Print and shaded views of the part. All mm, measured from the part's lowest x, y and z. A direction names the side the tool comes from. Round coordinates to 2 decimals unless told otherwise and drop trailing zeros. Loops run counter-clockwise (first coordinate to the right, second up) from the corner with the lowest first, then second, coordinate; pieces in that order, holes last. Notation, with made-up numbers: (11, -22) - (31, -22) arc R18 ccw to (31, -9) - close; hole circle Ø2 at (8, 1.5). An arc over 180 degrees is marked (long way). Answer as a JSON object with one key per item and string values.
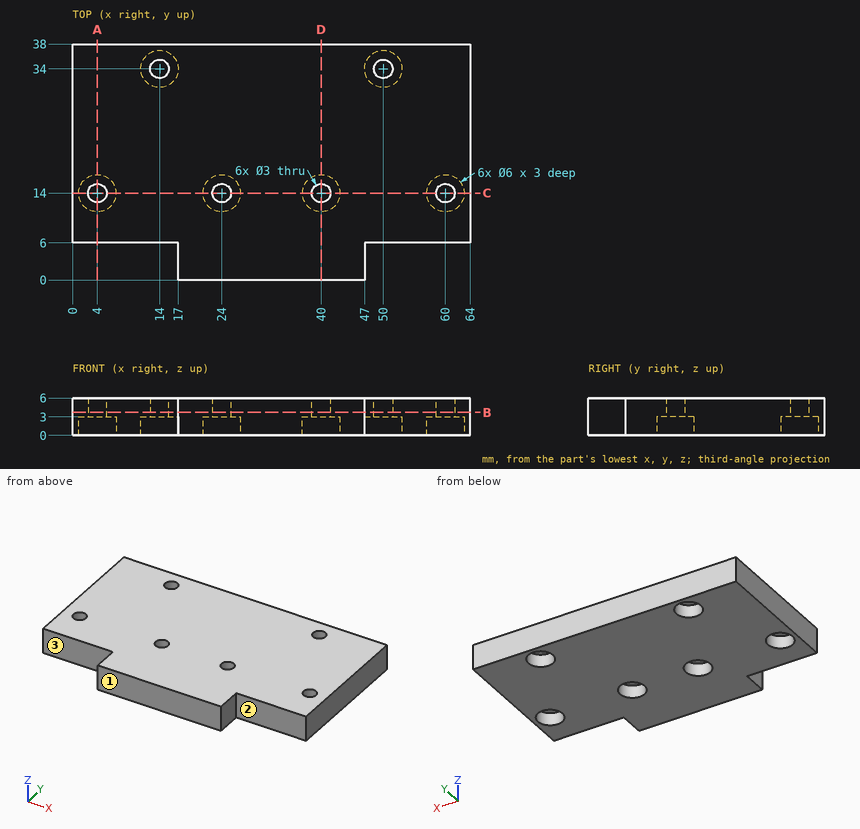
1) Tool access for the marked faces 1, 2 and 3: list every direction of +Z, -Z, +X, -X, +Y, -Y with a clear straight run to the whole face (end or side of a thin tool).
Values follow:
{"face 1": "+Z, -Z, +X, -X, -Y", "face 2": "+Z, -Z, +X, -Y", "face 3": "+Z, -Z, -X, -Y"}
2) Slice it at C-C on y = 14. Count the separate pieces of the cut face and the enclosed holes in it, then the cut area to 3 significant figures.
Values follow:
{"separate pieces": "5", "enclosed holes": "0", "area": "276 mm²"}
3) Drop flat-ended pins along their axis: P1, Ø3, axis at x = 10, z = 3, coming from the -Y side; P2, Ø3.5, axis at x = 50, y = 34, coming from the -Z side. Give the stop position or say it passes through.
Values follow:
{"P1": "y = 6", "P2": "z = 3"}
4) Probe probe 1 along Y at (x, z) = (40, 1.35); probe 2 along Y at (x, z) = (14, 5.35); probe 3 along Y at (x, z) = (11, 5.55). List the from-to ranges inside material, lowest first.
Values follow:
{"probe 1": "0 to 11, 17 to 38", "probe 2": "6 to 32.5, 35.5 to 38", "probe 3": "6 to 38"}
5) Slice it at B-B on z = 3.7. List the corners of the cut face in (x, y), then the cut area to 3 significant figures.
Values follow:
{"outline": "(0, 6) - (17, 6) - (17, 0) - (47, 0) - (47, 6) - (64, 6) - (64, 38) - (0, 38) - close; hole circle Ø3 at (4, 14); hole circle Ø3 at (14, 34); hole circle Ø3 at (24, 14); hole circle Ø3 at (40, 14); hole circle Ø3 at (50, 34); hole circle Ø3 at (60, 14)", "area": "2,190 mm²"}
6) Slice it at A-A on x = 4. List the corners of the cut face in (y, z), then the cut area to 3 significant figures.
Values follow:
{"outline": "(6, 0) - (11, 0) - (11, 3) - (12.5, 3) - (12.5, 6) - (6, 6) - close; (15.5, 3) - (17, 3) - (17, 0) - (38, 0) - (38, 6) - (15.5, 6) - close", "area": "165 mm²"}
7) Slice it at D-D on x = 40. List the corners of the cut face in (y, z).
Values follow:
{"outline": "(0, 0) - (11, 0) - (11, 3) - (12.5, 3) - (12.5, 6) - (0, 6) - close; (15.5, 3) - (17, 3) - (17, 0) - (38, 0) - (38, 6) - (15.5, 6) - close"}
